from build123d import *
from build123d.topology import SkipClean

# Parameters (mm, degrees)
SKETCH1_R           = 28
SKETCH1_R_2         = 2
BOSS_EXTRUDE1_DEPTH = 32
SKETCH2_R           = 24
CUT_EXTRUDE1_DEPTH  = 20
CUT_EXTRUDE2_DEPTH  = 4
CUT_EXTRUDE4_DEPTH  = 51.911688245


with BuildPart() as part:
    # Sketch1 → Boss-Extrude1 (new body)
    with BuildSketch(Plane.XY):
        Circle(SKETCH1_R)
        Circle(SKETCH1_R_2, mode=Mode.SUBTRACT)
    extrude(amount=BOSS_EXTRUDE1_DEPTH)

    # Sketch2 → Cut-Extrude1 (cut)
    with BuildSketch(Plane(origin=(0, 0, 0), x_dir=(-1, 0, 0), z_dir=(0, 0, -1))):
        Circle(SKETCH2_R)
    extrude(amount=-CUT_EXTRUDE1_DEPTH, mode=Mode.SUBTRACT)

    # Sketch3 → Cut-Extrude2 (cut)
    with BuildSketch(Plane(origin=(0, 0, 20), x_dir=(-1, 0, 0), z_dir=(0, 0, -1))):
        Polygon((6, 0), (3, 5.196152423), (-3, 5.196152423), (-6, 0), (-3, -5.196152423), (3, -5.196152423), align=None)
    extrude(amount=-CUT_EXTRUDE2_DEPTH, mode=Mode.SUBTRACT)

    # Sketch5 → Cut-Extrude4 (cut, through all)
    with SkipClean():  # the faces are left unmerged after this step: merging them gives an invalid solid
        with BuildSketch(Plane.XY.offset(32)):
            with BuildLine():
                Line((-7, 22.956480566), (-2, 6.708203932))
                ThreePointArc((-2, 6.708203932), (0, 7), (2, 6.708203932))
                Line((2, 6.708203932), (7, 22.956480566))
                ThreePointArc((7, 22.956480566), (0, 24), (-7, 22.956480566))
            make_face()
            with BuildLine():
                Line((13.583670621, 19.785951897), (3.997705422, 5.746159706))
                ThreePointArc((3.997705422, 5.746159706), (5.472820377, 4.364428613), (6.491664629, 2.618833776))
                Line((6.491664629, 2.618833776), (22.312527847, 8.840311143))
                ThreePointArc((22.312527847, 8.840311143), (18.763955579, 14.963755245), (13.583670621, 19.785951897))
            make_face()
            with BuildLine():
                Line((23.938560207, 1.716197889), (6.985057122, 0.45714002))
                ThreePointArc((6.985057122, 0.45714002), (6.824495385, -1.557646538), (6.094973386, -3.442571629))
                Line((6.094973386, -3.442571629), (20.823267132, -11.932792881))
                ThreePointArc((20.823267132, -11.932792881), (23.398269892, -5.340502415), (23.938560207, 1.716197889))
            make_face()
            with BuildLine():
                Line((16.2672257, -17.645888133), (4.712518341, -5.176115424))
                ThreePointArc((4.712518341, -5.176115424), (3.037186174, -6.306782075), (1.108642869, -6.911650381))
                Line((1.108642869, -6.911650381), (3.65366155, -23.720260481))
                ThreePointArc((3.65366155, -23.720260481), (10.413209739, -21.62325283), (16.2672257, -17.645888133))
            make_face()
            with BuildLine():
                Line((-3.65366155, -23.720260481), (-1.108642869, -6.911650381))
                ThreePointArc((-1.108642869, -6.911650381), (-3.037186174, -6.306782075), (-4.712518341, -5.176115424))
                Line((-4.712518341, -5.176115424), (-16.2672257, -17.645888133))
                ThreePointArc((-16.2672257, -17.645888133), (-10.413209739, -21.62325283), (-3.65366155, -23.720260481))
            make_face()
            with BuildLine():
                Line((-20.823267132, -11.932792881), (-6.094973386, -3.442571629))
                ThreePointArc((-6.094973386, -3.442571629), (-6.824495385, -1.557646538), (-6.985057122, 0.45714002))
                Line((-6.985057122, 0.45714002), (-23.938560207, 1.716197889))
                ThreePointArc((-23.938560207, 1.716197889), (-23.398269892, -5.340502415), (-20.823267132, -11.932792881))
            make_face()
            with BuildLine():
                Line((-22.312527847, 8.840311143), (-6.491664629, 2.618833776))
                ThreePointArc((-6.491664629, 2.618833776), (-5.472820377, 4.364428613), (-3.997705422, 5.746159706))
                Line((-3.997705422, 5.746159706), (-13.583670621, 19.785951897))
                ThreePointArc((-13.583670621, 19.785951897), (-18.763955579, 14.963755245), (-22.312527847, 8.840311143))
            make_face()
        extrude(amount=-CUT_EXTRUDE4_DEPTH, mode=Mode.SUBTRACT)


solid = part.part
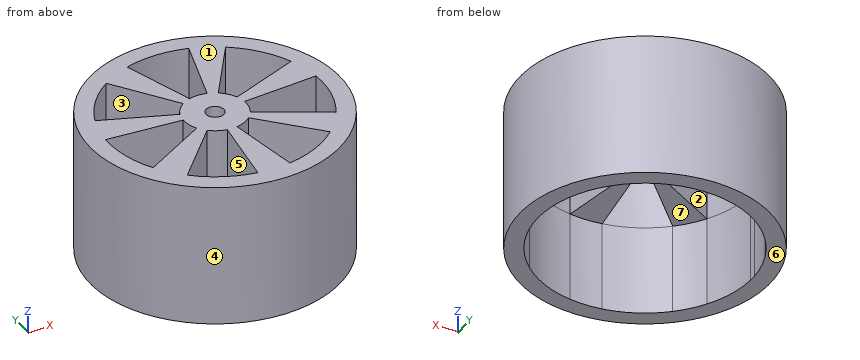
Input: part model. Units: mm. Frame: model coordinates. Face numbers are marked on the shaded views. A direction names the side the tool comes from. Round coordinates to 2 decimals unless told otherwise and drop trailing zeros. Loops run counter-clockwise (first coordinate to the right, second up) from the corner with the lowest first, then second, coordinate; pieces in that order, holes last. Notation, with made-up numbers: (-23, 80.25) -> (8, 80.25) arc R18 cw to (8, 95.25) -> close; hole circle Ø2 at (-12, -1). An arc over 180 degrees is marked (long way). Answer as a JSON object with one key per item and string values. Group by question number.
1) Reachability of the marked faces 5, 6 and 7 from +Z, -Z, +X, -X, +Y, -Y: full face, straight path, thin tool, end or side. Return the list, or none.
2) Section query A-A on y = -9. Output: boundary loops of the cut face in (x, z).
3) Section query B-B on x = 0. Output: boundary loops of the cut face in (y, z), plus the area to 3 significant figures.
4) Draft query along Y for the marked faces 1, 2, 3 and 4. Return one class per face: +Y half, -Y half, draft (parallel to the pull), parting line (faces both ways), or undercut.
5) Section query D-D on x = -12. Output: boundary loops of the cut face in (y, z), plus the area to 3 significant figures.
6) Section query C-C on y = -21. Output: boundary loops of the cut face in (x, z), plus the area to 3 significant figures.
7) Ray query, L1, parallel to Y at x = 0, z = 28; L2, parallel to X at y = -1, z = 26; L3, parallel to X at y = -15, z = 29.5. Return the intervals inside material, ascending.
8) Pin query (flat end, axial travel): pin 1 (1.2 mm diameter, centred on x = 1, z = 21.5, fed in from +Y); pin 2 (1 mm diameter, centred on y = 17, z = 7, fed in from +X); pin 3 (4.5 mm diameter, centred on x = 1.5, z = 21, fed in from -Y); pin 4 (3.5 mm diameter, centred on x = 0, y = 0, fed in from +Z). Return the tip coordinate at first contact, or that it passes through.
Reply:
{
 "1": {"face 5": "+Z, -Z", "face 6": "-Z, +X, -X, +Y, -Y", "face 7": "-Z"},
 "2": {"outline": "(-26.51, 0) -> (-22.25, 0) -> (-22.25, 32) -> (-26.51, 32) -> close; (-15.74, 20) -> (-8.26, 20) -> (-8.26, 32) -> (-15.74, 32) -> close; (-1.42, 20) -> (1.42, 20) -> (1.42, 32) -> (-1.42, 32) -> close; (8.26, 20) -> (15.74, 20) -> (15.74, 32) -> (8.26, 32) -> close; (22.25, 0) -> (26.51, 0) -> (26.51, 32) -> (22.25, 32) -> close"},
 "3": {"outline": "(-28, 0) -> (-24, 0) -> (-24, 20) -> (-5.2, 20) -> (-5.2, 24) -> (-2, 24) -> (-2, 32) -> (-28, 32) -> close; (2, 24) -> (5.2, 24) -> (5.2, 20) -> (7, 20) -> (7, 32) -> (2, 32) -> close; (24, 0) -> (28, 0) -> (28, 32) -> (24, 32) -> close", "area": "554 mm2"},
 "4": {"face 1": "draft", "face 2": "undercut", "face 3": "undercut", "face 4": "parting line"},
 "5": {"outline": "(-25.3, 0) -> (-20.78, 0) -> (-20.78, 32) -> (-25.3, 32) -> close; (-13.04, 20) -> (-6.85, 20) -> (-6.85, 32) -> (-13.04, 32) -> close; (0.83, 20) -> (4.78, 20) -> (4.78, 32) -> (0.83, 32) -> close; (17.47, 20) -> (20.78, 20) -> (20.78, 0) -> (25.3, 0) -> (25.3, 32) -> (17.47, 32) -> close", "area": "450 mm2"},
 "6": {"outline": "(-18.52, 0) -> (-11.62, 0) -> (-11.62, 32) -> (-18.52, 32) -> close; (-3.24, 20) -> (3.24, 20) -> (3.24, 32) -> (-3.24, 32) -> close; (11.62, 0) -> (18.52, 0) -> (18.52, 32) -> (11.62, 32) -> close", "area": "519 mm2"},
 "7": {"L1": "y = -28 to -2, 2 to 7, 24 to 28", "L2": "x = -27.98 to -23.98, -6.93 to -1.73, 1.73 to 6.93, 23.98 to 27.98", "L3": "x = -23.64 to -13.82, -2.33 to 2.33, 13.82 to 23.64"},
 "8": {"pin 1": "stops at y = 28", "pin 2": "stops at x = 22.62", "pin 3": "stops at y = -28", "pin 4": "passes through"}
}
